Could you check a few things on this model? Use its own coordinates, in mm. Face numbers are marked on the shaded views. A direction names the side the tool comes from. Coordinates: 2 decimals unless noted, no trailing zeros. Order: outer loops, then holes, each group sorted by start corner. A loop starts at its lowest first (then second) coordinate and runs counter-clockwise, first axis right, second up. Notation, with made-up numbers: (-36, 38.5) - (-28, 38.5) arc R15 ccw to (-28, 56.5) - close; hole circle Ø3 at (82, -3.75). An arc over 180 degrees is marked (long way). Answer as a JSON object with one key per item and string values. Group by question number.
(1) Will these pins go through, and if not, where does the flat tip stop? P1, Ø10, axis at y = -8, z = 39, coming from the -X side; P2, Ø1.5, axis at x = 25.5, z = 27.5, coming from the +Y side; P3, Ø16, axis at x = -61.98, z = 30.9, coming from the -Y side.
(2) Imagine slicing it at B-B, the plane x = 73.5. Write out the boundary of the cut face in (y, z).
(3) Please list where these lines run through material, in increasing order: probe 1 along Z at (x, y) = (-23, -44.5); probe 2 along X at (y, z) = (-9.5, 22); probe 3 along X at (y, z) = (-14, 26.5).
(4) Imagine slicing it at D-D, the plane y = -30.5. Give the number of separate pieces and of enclosed holes in the cut face, and give its area (3 significant figures).
(5) We'd pull the mould along X, two halves only. Please class the marked faces 3, 4 and 5: pulls with the +X half, pulls with the -X half, needs draft (parallel to the pull), parting line crosses it, or undercut.
(6) Imagine slicing it at C-C, the plane x = 15.5. Write out the boundary of the cut face in (y, z).
(7) Which directions (+Z, -Z, +X, -X, +Y, -Y) give clear straight access to the entire face, cutting with the end or side of a thin tool? Please do the marked faces 1 and 2.
(8) Imagine slicing it at A-A, the plane z = 37. Write out the boundary of the cut face in (x, y), and give its area (3 significant figures).
from build123d import *

# Parameters (mm, degrees)
F0_R     = 12.5
F0_R_2   = 9.5
F3_T     = -2.5
F5_START = 27.9
F5_DEPTH = 70.8


with BuildPart() as f2:
    # F2: sweep along a path in F1
    with BuildLine(Plane.XY) as f2_path:
        Line((-30.2034914494, 0), (-30.2034914494, -12))
        ThreePointArc((-30.2034914494, -12), (-27.2745592612, -19.0710678119), (-20.2034914494, -22))
        Line((-20.2034914494, -22), (44.7965085506, -22))
    # F0 (on Front) → F2 (sweep)
    with BuildSketch(Plane.XZ):
        with Locations((-61.9814805686, 30.9009179473)):
            Circle(F0_R)
        with Locations((-61.9814805686, 30.9009179473)):
            Circle(F0_R_2, mode=Mode.SUBTRACT)
        with Locations((-61.9814805686, 30.9009179473)):
            Circle(F0_R_2)
    sweep(path=f2_path.line)

    # F3
    f3_openings = [f2.faces().sort_by_distance(p)[0] for p in [
        (44.796509, -53.777989, 30.900918),
        (-61.981481, 0, 30.900918),
    ]]
    offset(amount=F3_T, openings=f3_openings)

    # F4 (on Right) → F5 (join)
    with BuildSketch(Plane.YZ.offset(F5_START)):
        with BuildLine():
            Line((-53.509484202, 46.3802992553), (-51.3534231177, 46.3802992553))
            ThreePointArc((-51.3534231177, 46.3802992553), (-52.4314536598, 46.4178383598), (-53.509484202, 46.3802992553))
        make_face()
        with BuildLine():
            Line((-36.3746711443, 46.3802992553), (-51.3534231177, 46.3802992553))
            Line((-51.3534231177, 46.3802992553), (-53.509484202, 46.3802992553))
            ThreePointArc((-53.509484202, 46.3802992553), (-67.929370479, 30.8835584681), (-53.4370074848, 15.4545756724))
            Line((-53.4370074848, 15.4545756724), (-36.3746711443, 15.7140511985))
            Line((-36.3746711443, 15.7140511985), (-36.3746711443, 46.3802992553))
        make_face()
        with BuildLine():
            ThreePointArc((-54.6600517166, 41.3802992553), (-53.4043908119, 41.4556498275), (-52.1487299073, 41.3802992553))
            Line((-52.1487299073, 41.3802992553), (-41.3746711443, 41.3802992553))
            Line((-41.3746711443, 41.3802992553), (-41.3746711443, 20.6385918219))
            Line((-41.3746711443, 20.6385918219), (-53.0851070952, 20.4605053354))
            ThreePointArc((-53.0851070952, 20.4605053354), (-53.2447304946, 20.4568637746), (-53.4043908119, 20.4556498275))
            ThreePointArc((-53.4043908119, 20.4556498275), (-63.8855362405, 30.3266899686), (-54.6600517166, 41.3802992553))
        make_face(mode=Mode.SUBTRACT)
    extrude(amount=F5_DEPTH)

    # F6: sweep along a path in F1
    with BuildLine(Plane.XY) as f6_path:
        Line((-30.2034914494, 0), (-30.2034914494, -12))
        ThreePointArc((-30.2034914494, -12), (-27.2745592612, -19.0710678119), (-20.2034914494, -22))
        Line((-20.2034914494, -22), (44.7965085506, -22))
    # F4 (on Right) → F6 (sweep)
    with BuildSketch(Plane.YZ):
        with BuildLine():
            Line((-36.3746711443, 46.3802992553), (-51.3534231177, 46.3802992553))
            Line((-51.3534231177, 46.3802992553), (-53.509484202, 46.3802992553))
            ThreePointArc((-53.509484202, 46.3802992553), (-67.929370479, 30.8835584681), (-53.4370074848, 15.4545756724))
            Line((-53.4370074848, 15.4545756724), (-36.3746711443, 15.7140511985))
            Line((-36.3746711443, 15.7140511985), (-36.3746711443, 46.3802992553))
        make_face()
        with BuildLine():
            ThreePointArc((-54.6600517166, 41.3802992553), (-53.4043908119, 41.4556498275), (-52.1487299073, 41.3802992553))
            Line((-52.1487299073, 41.3802992553), (-41.3746711443, 41.3802992553))
            Line((-41.3746711443, 41.3802992553), (-41.3746711443, 20.6385918219))
            Line((-41.3746711443, 20.6385918219), (-53.0851070952, 20.4605053354))
            ThreePointArc((-53.0851070952, 20.4605053354), (-53.2447304946, 20.4568637746), (-53.4043908119, 20.4556498275))
            ThreePointArc((-53.4043908119, 20.4556498275), (-63.8855362405, 30.3266899686), (-54.6600517166, 41.3802992553))
        make_face(mode=Mode.SUBTRACT)
    sweep(path=f6_path.line)


solid = f2.part
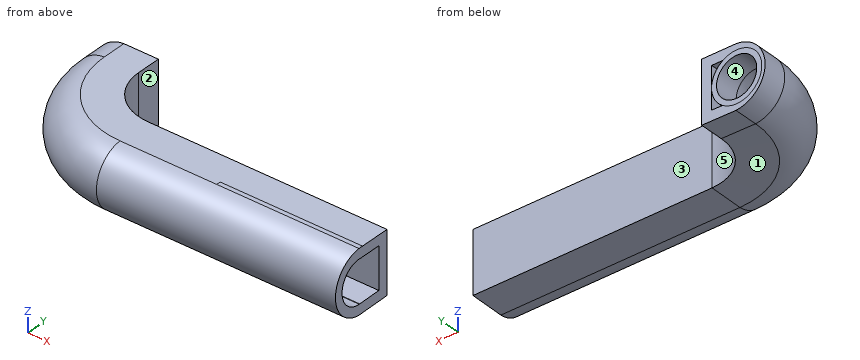
Result set:
{
 "1": {"P1": "stops at x = -75.82", "P2": "stops at y = -36.37", "P3": "stops at y = -56.58"},
 "2": {"outline": "(-53.44, 15.45) - (-36.37, 15.71) - (-36.37, 46.38) - (-51.35, 46.38) arc R15.5 ccw to start; hole (-53.09, 20.46) - (-41.37, 20.64) - (-41.37, 41.38) - (-52.15, 41.38) arc R10.5 ccw (long way) to start"},
 "3": {"probe 1": "z = 15.59 to 20.59, 22.39 to 26.88, 34.92 to 39.41, 41.38 to 46.38", "probe 2": "x = -73.31 to -66.54, -57.42 to -53.21, -49.58 to -44.58", "probe 3": "x = -75.45 to -70.92, -52.94 to -50.22, -49.51 to -44.5"},
 "4": {"separate pieces": "1", "enclosed holes": "3", "area": "636 mm^2"},
 "5": {"face 3": "needs draft", "face 4": "undercut", "face 5": "pulls with the +X half"},
 "6": {"outline": "(-53.51, 46.38) arc R15.5 ccw to (-53.44, 15.45) - (-36.37, 15.71) - (-36.37, 46.38) - close; hole circle Ø20 at (-53.78, 30.9); hole (-46.96, 41.38) arc R12.5 cw to (-41.37, 32.45) - (-41.37, 41.38) - close; hole (-46.76, 20.56) - (-41.37, 20.64) - (-41.37, 29.35) arc R12.5 cw to start"},
 "7": {"face 1": "-Z, +X, +Y", "face 2": "+Z, -Z, +X, +Y"},
 "8": {"outline": "(-74.89, -12) arc R54.69 ccw to (-20.2, -66.69) - (98.7, -66.69) - (98.7, -61.99) - (44.8, -61.99) - (44.8, -61.7) - (-20.2, -61.7) arc R49.7 cw to (-69.91, -12) - (-69.91, 0) - (-74.89, 0) - close; (-54.06, -12) arc R33.85 ccw to (-20.2, -45.85) - (44.8, -45.85) - (44.8, -42.87) - (-20.2, -42.87) arc R30.87 cw to (-51.07, -12) - (-51.07, 0) - (-54.06, 0) - close; (-49.58, -12) arc R29.37 ccw to (-20.2, -41.37) - (98.7, -41.37) - (98.7, -36.37) - (-20.2, -36.37) arc R24.37 cw to (-44.58, -12) - (-44.58, 0) - (-49.58, 0) - close", "area": "2,290 mm^2"}
}
